Study the drawing (mm; zero at the part's minimum x, y, z) and answer. Coordinates: 2 decimals unless noted, no trailing zeros. Order: outer loops, then holes, each group sorted by start corner. A loop starts at its lowest first (then second) coordinate and runs counter-clockwise, first axis right, second up. Notation, with made-up numbers: M 82,38.25 L 101,38.25 A25 cw 101,70.25 Z; hole C 5.25,9 d8. An arc over 180 degrees is marked long. One line per item, written item: value. Start each with the question number.
Q1. The part is cut by section C-C on z = 6. Give the vertices of the cut face in (x, y).
Q2. The part is cut by section A-A on y = 20. Give the vertices of the cut face in (x, z), then the cut area to 3 significant figures.
Q3. The part is cut by section D-D on y = 28. Give the vertices of the cut face in (x, z).
Q4. Each of these flat-tipped pins is pushed along its axis until it touches: pin 1 Ø3 at (x, y) = (20, 12) entering from +Z; pin 2 Ø3 at (x, z) = (16.5, 2.5) entering from -Y; pin 3 Ø1 at (x, z) = (7.5, 5.5) entering from +Y; pin 4 Ø2 at (x, z) = (32, 3.5) entering from -Y. Where does it stop, or does it pass through?
Q5. Determine the mould class of the marked faces 1, 2 and 3 for opening direction X: pulls with the +X half, pulls with the -X half, needs draft (parallel to the pull), parting line crosses it, or undercut.
Q6. Straight lines are drawn through the part: line 1 along Y through (x, z) = (20, 3.5); line 2 along X through (y, z) = (20.5, 1); line 3 along Y through (x, z) = (27, 0.5) (3 decimals). For each, find the intervals that lie inside material, in ascending order. Write a range as [from, to].
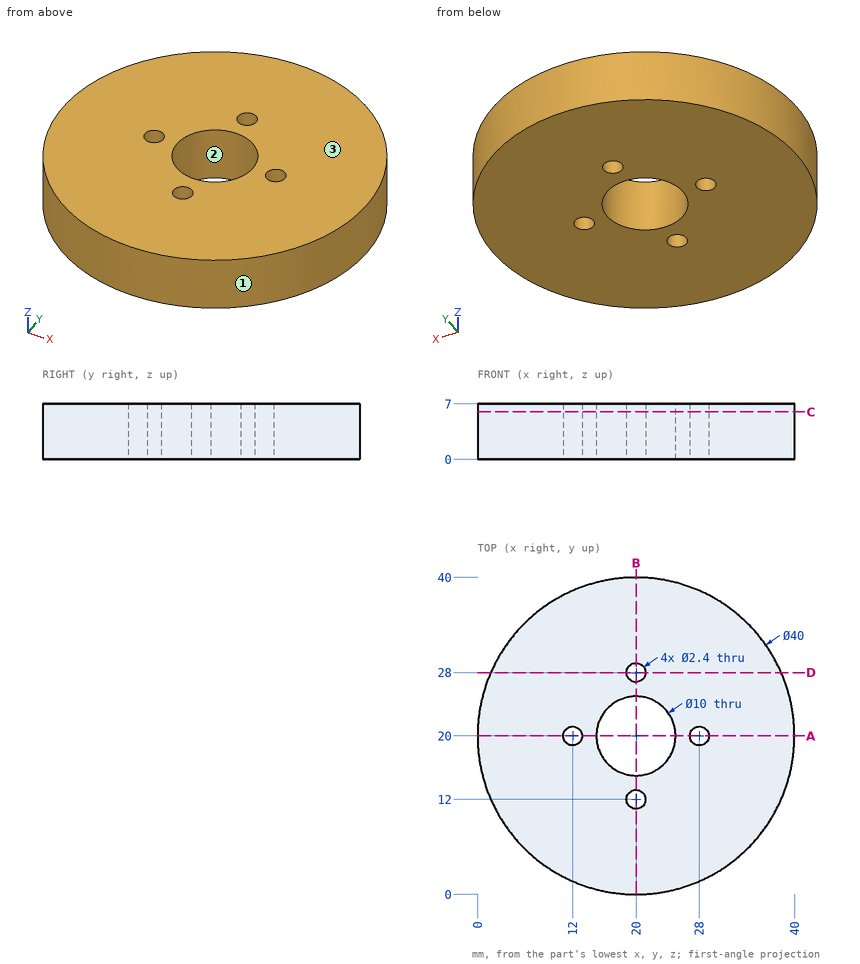
Output:
1. outline: C 20,20 d40; hole C 12,20 d2.4; hole C 20,20 d10; hole C 20,12 d2.4; hole C 20,28 d2.4; hole C 28,20 d2.4
2. outline: M 0,0 L 10.8,0 L 10.8,7 L 0,7 Z; M 13.2,0 L 15,0 L 15,7 L 13.2,7 Z; M 25,0 L 26.8,0 L 26.8,7 L 25,7 Z; M 29.2,0 L 40,0 L 40,7 L 29.2,7 Z
2. area: 176 mm^2
3. outline: M 1.67,0 L 18.8,0 L 18.8,7 L 1.67,7 Z; M 21.2,0 L 38.33,0 L 38.33,7 L 21.2,7 Z
4. pin 1: stops at z = 7
4. pin 2: stops at y = 0.1
4. pin 3: stops at y = 36
4. pin 4: stops at y = 3.3
5. face 1: parting line crosses it
5. face 2: undercut
5. face 3: needs draft
6. line 1: y = [0, 10.8], [13.2, 15], [25, 26.8], [29.2, 40]
6. line 2: x = [0.01, 10.91], [13.09, 15.03], [24.97, 26.91], [29.09, 39.99]
6. line 3: y = [1.265, 19.337], [20.663, 38.735]
